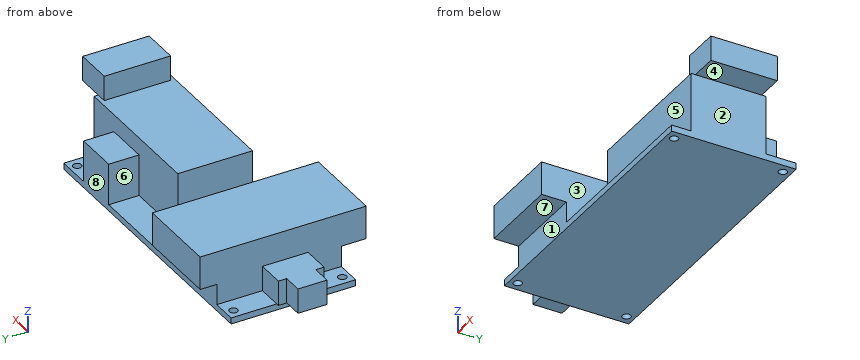
from build123d import *

# Parameters (mm, degrees)
SKETCH002_W  = 70
SKETCH002_H  = 30
SKETCH002_R  = 1
PAD002_DEPTH = 1.5
SKETCH003_W  = 20
SKETCH003_H  = 30
PAD003_DEPTH = 5
SKETCH004_W  = 20
SKETCH004_H  = 40
PAD004_DEPTH = 8
SKETCH005_W  = 35
SKETCH005_H  = 18
PAD005_DEPTH = 14.2
SKETCH006_W  = 9
SKETCH006_H  = 16
PAD006_DEPTH = 6
SKETCH010_W  = 10.5
SKETCH010_H  = 7.3
PAD009_DEPTH = 10
PAD010_DEPTH = 6


with BuildPart() as part:
    # Sketch002 → Pad002 (new body)
    with BuildSketch(Plane.XY):
        Rectangle(SKETCH002_W, SKETCH002_H)
        with Locations((-32.7, 13.1)):
            Circle(SKETCH002_R, mode=Mode.SUBTRACT)
        with Locations((-32.7, -13.1)):
            Circle(SKETCH002_R, mode=Mode.SUBTRACT)
        with Locations((32.7, 13.1)):
            Circle(SKETCH002_R, mode=Mode.SUBTRACT)
        with Locations((32.7, -13.1)):
            Circle(SKETCH002_R, mode=Mode.SUBTRACT)
    extrude(amount=PAD002_DEPTH)

    # Sketch003 (on Face10 of Pad002) → Pad003 (join)
    with BuildSketch(Plane.XY.offset(1.5)):
        with Locations((-19, 0)):
            Rectangle(SKETCH003_W, SKETCH003_H)
    extrude(amount=PAD003_DEPTH)

    # Sketch004 (on Face15 of Pad003) → Pad004 (join)
    with BuildSketch(Plane.XY.offset(6.5)):
        with Locations((-19, -1)):
            Rectangle(SKETCH004_W, SKETCH004_H)
    extrude(amount=PAD004_DEPTH)

    # Sketch005 (on Face13 of Pad004) → Pad005 (join)
    with BuildSketch(Plane.XY.offset(1.5)):
        with Locations((17.5, -1.3)):
            Rectangle(SKETCH005_W, SKETCH005_H)
    extrude(amount=PAD005_DEPTH)

    # Sketch006 (on Face27 of Pad005) → Pad006 (join)
    with BuildSketch(Plane.XY.offset(15.7)):
        with Locations((37, -1.3)):
            Rectangle(SKETCH006_W, SKETCH006_H)
    extrude(amount=PAD006_DEPTH)

    # Sketch010 (on Face13 of Pad006) → Pad009 (join)
    with BuildSketch(Plane.XY.offset(1.5)):
        with Locations((21.45, 11.35)):
            Rectangle(SKETCH010_W, SKETCH010_H)
    extrude(amount=PAD009_DEPTH)

    # Sketch012 (on Face12 of Pad009) → Pad010 (join)
    with BuildSketch(Plane.XY.offset(1.5)):
        Polygon((-29, 4), (-35.7, 4), (-35.7, 2), (-40.4, 2), (-40.4, -5), (-35.7, -5), (-35.7, -7), (-29, -7), align=None)
    extrude(amount=PAD010_DEPTH)


with BuildPart() as part_1:
    # Body001 placement: moved
    add(part.part.moved(Location((0, -19.6, 4))))


solid = part_1.part
Part model, mm, in its own coordinate system. Face numbers are marked on the shaded views. A direction names the side the tool comes from. Give positions to 0.01 mm unless a question says otherwise; leave off trailing zeros. Write each loop counter-clockwise with the first axis right and the second up, starting at its lowest first coordinate (ties: lowest second). Pieces come first, ordered by that corner, then holes.
1) Probe L1, parallel to Y at x = 32.7, z = 4.4; L2, parallel to X at y = -20, z = 13.5; L3, parallel to X at y = -23, z = 9. List the from-to ranges inside material, lowest first.
Resolved:
L1: y = -34.6 to -33.7, -31.7 to -7.5, -5.5 to -4.6
L2: x = -29 to -9, 0 to 35
L3: x = -40.4 to -9, 0 to 35
2) Cut at A-A on x = -32.7. Write the cut outline in (y, z), then the cut area to 3 significant figures.
Resolved:
outline: (-34.6, 4) - (-33.7, 4) - (-33.7, 5.5) - (-34.6, 5.5) - close; (-31.7, 4) - (-7.5, 4) - (-7.5, 5.5) - (-15.6, 5.5) - (-15.6, 11.5) - (-26.6, 11.5) - (-26.6, 5.5) - (-31.7, 5.5) - close; (-5.5, 4) - (-4.6, 4) - (-4.6, 5.5) - (-5.5, 5.5) - close
area: 105 mm2
3) Cut at B-B on y = -6.5. Write the cut outline in (x, z), then the cut area to 3 significant figures.
Resolved:
outline: (-35, 4) - (-33.7, 4) - (-33.7, 5.5) - (-35, 5.5) - close; (-31.7, 4) - (31.7, 4) - (31.7, 5.5) - (26.7, 5.5) - (26.7, 15.5) - (16.2, 15.5) - (16.2, 5.5) - (-9, 5.5) - (-9, 18.5) - (-29, 18.5) - (-29, 5.5) - (-31.7, 5.5) - close; (33.7, 4) - (35, 4) - (35, 5.5) - (33.7, 5.5) - close
area: 464 mm2
4) Two-plate mould, pull along X, no slides. Class the marked faces 1, 2 and 3: released by +X, released by -X, zero draft, split by the parting line, or undercut.
Resolved:
face 1: zero draft
face 2: released by +X
face 3: undercut
5) Pin check, flat tips, straight feed: pin 1 (2 mm diameter, centred on x = 7.5, y = -9.5, fed in from +Z); pin 2 (8 mm diameter, centred on x = 6.5, z = 21.5, fed in from +Y); pin 3 (8 mm diameter, centred on x = 21.5, y = -6.5, fed in from +Z). Stop position of each tip, or through.
Resolved:
pin 1: stops at z = 5.5
pin 2: stops at y = -11.9
pin 3: stops at z = 15.5
6) Cut at C-C on y = -20. Write the cut outline in (x, z), then the cut area to 3 significant figures.
Resolved:
outline: (-40.4, 5.5) - (-35, 5.5) - (-35, 4) - (35, 4) - (35, 19.7) - (41.5, 19.7) - (41.5, 25.7) - (32.5, 25.7) - (32.5, 19.7) - (0, 19.7) - (0, 5.5) - (-9, 5.5) - (-9, 18.5) - (-29, 18.5) - (-29, 11.5) - (-40.4, 11.5) - close
area: 984 mm2
7) Which spindle directions (+Z, -Z, +X, -X, +Y, -Y) get a long thin tool onto all of the face, cutting with end or side? Do the marked faces 4, 5, 6, 7 and 8. Say none if no direction does.
Resolved:
face 4: -Z, +X, +Y, -Y
face 5: +Z, +X, -Y
face 6: +Z, +Y
face 7: -Z, +X, -X, -Y
face 8: -Z, +X, +Y
8) Cut at D-D on x = -21.5. Write the cut outline in (y, z), then the cut area to 3 significant figures.
Resolved:
outline: (-40.6, 10.5) - (-34.6, 10.5) - (-34.6, 4) - (-4.6, 4) - (-4.6, 10.5) - (-0.6, 10.5) - (-0.6, 18.5) - (-40.6, 18.5) - close
area: 515 mm2
